from build123d import *

# Parameters (mm, degrees)
SKETCH_2_W                = 72
SKETCH_2_H                = 64
SKETCH_2_R                = 2.25
SKETCH_2_R_2              = 1.75
EXTRUDE_1_DEPTH           = 7
HOLE_WIZARD_1_D           = 4.5
HOLE_WIZARD_1_CBORE_D     = 7.3
HOLE_WIZARD_1_CBORE_DEPTH = 4.2
CUT_EXTRUDE_1_DEPTH       = 2.5


with BuildPart() as part:
    # 草圖2 → 填料-伸長1 (new body)
    with BuildSketch(Plane.XY):
        Rectangle(SKETCH_2_W, SKETCH_2_H)
        with Locations((-18, 18)):
            Circle(SKETCH_2_R, mode=Mode.SUBTRACT)
        with Locations((-31, 26)):
            Circle(SKETCH_2_R_2, mode=Mode.SUBTRACT)
        with Locations((18, 18)):
            Circle(SKETCH_2_R, mode=Mode.SUBTRACT)
        with Locations((18, -18)):
            Circle(SKETCH_2_R, mode=Mode.SUBTRACT)
        with Locations((-18, -18)):
            Circle(SKETCH_2_R, mode=Mode.SUBTRACT)
        with Locations((31, 26)):
            Circle(SKETCH_2_R_2, mode=Mode.SUBTRACT)
        with Locations((31, -26)):
            Circle(SKETCH_2_R_2, mode=Mode.SUBTRACT)
        with Locations((-31, -26)):
            Circle(SKETCH_2_R_2, mode=Mode.SUBTRACT)
    extrude(amount=EXTRUDE_1_DEPTH)

    # 鑽孔1 (through all)
    with Locations(Plane(origin=(-18, 18, 7), x_dir=(1, 0, 0), z_dir=(0, 0, 1))):
        with Locations((0, 0), (36, 0), (36, -36), (0, -36)):
            CounterBoreHole(HOLE_WIZARD_1_D / 2, HOLE_WIZARD_1_CBORE_D / 2, HOLE_WIZARD_1_CBORE_DEPTH)

    # 草圖4 → 除料-伸長1 (cut)
    with BuildSketch(Plane(origin=(0, 0, 0), x_dir=(-1, 0, 0), z_dir=(0, 0, -1))):
        Polygon((-27.709103466, 26), (-29.354551733, 28.85), (-32.645448267, 28.85), (-34.290896534, 26), (-32.645448267, 23.15), (-29.354551733, 23.15), align=None)
        Polygon((29.354551733, 23.15), (27.709103466, 26), (29.354551733, 28.85), (32.645448267, 28.85), (34.290896534, 26), (32.645448267, 23.15), align=None)
        Polygon((27.709103466, -26), (29.354551733, -28.85), (32.645448267, -28.85), (34.290896534, -26), (32.645448267, -23.15), (29.354551733, -23.15), align=None)
        Polygon((-29.354551733, -23.15), (-27.709103466, -26), (-29.354551733, -28.85), (-32.645448267, -28.85), (-34.290896534, -26), (-32.645448267, -23.15), align=None)
    extrude(amount=-CUT_EXTRUDE_1_DEPTH, mode=Mode.SUBTRACT)


solid = part.part
The model under review builds one solid part; all positions refer to its coordinate system, in mm. A direction names the side the tool comes from. Round coordinates to 2 decimals unless told otherwise and drop trailing zeros. Write each loop counter-clockwise with the first axis right and the second up, starting at its lowest first coordinate (ties: lowest second). Pieces come first, ordered by that corner, then holes. Notation, with made-up numbers: (75, -17.5) -> (89, -17.5) arc R15 ccw to (89, -1.5) -> close; hole circle Ø8 at (61.5, 3). An arc over 180 degrees is marked (long way). Answer as a JSON object with one key per item and string values.
1. We need section B-B on x = 31. State the section outline as (y, z) points.
Results found:
{"outline": "(-32, 0) -> (-28.85, 0) -> (-28.85, 2.5) -> (-27.75, 2.5) -> (-27.75, 7) -> (-32, 7) -> close; (-24.25, 2.5) -> (-23.15, 2.5) -> (-23.15, 0) -> (23.15, 0) -> (23.15, 2.5) -> (24.25, 2.5) -> (24.25, 7) -> (-24.25, 7) -> close; (27.75, 2.5) -> (28.85, 2.5) -> (28.85, 0) -> (32, 0) -> (32, 7) -> (27.75, 7) -> close"}
2. The part is to be moulded in two halves that separate along Y. For faces 1 (the face through (-1, 0, 0)), 2 (the face through (29.71, -24.82, 4.72)), say which applies: pulls with the +Y half, pulls with the -Y half, needs draft (parallel to the pull), parting line crosses it, or undercut.
Results found:
{"face 1": "needs draft", "face 2": "undercut"}
3. To check wall thickness, follow line 1 along Y through (x, z) = (18, 5); line 2 along Y through (x, z) = (-31, 5.35); line 3 along X through (y, z) = (-27, 5). State the ranges of each line that lie inside material, in increasing order.
Results found:
{"line 1": "y = -32 to -21.65, -14.35 to 14.35, 21.65 to 32", "line 2": "y = -32 to -27.75, -24.25 to 24.25, 27.75 to 32", "line 3": "x = -36 to -32.44, -29.56 to 29.56, 32.44 to 36"}
4. We need section C-C on z = 1. State how many separate pieces and enclosed holes the cut face has, and give its area (3 significant figures).
Results found:
{"separate pieces": "1", "enclosed holes": "8", "area": "4,430 mm^2"}
5. Clearance check with flat-ended pins moving along their axes: pin 1 (5 mm diameter, centred on x = -18, y = -18, fed in from +Z); pin 2 (2 mm diameter, centred on x = -17.5, y = -18.5, fed in from +Z); pin 3 (4.5 mm diameter, centred on x = -31, y = -26, fed in from -Z). State where each tip first meets the part, or that it passes through.
Results found:
{"pin 1": "stops at z = 2.8", "pin 2": "passes through", "pin 3": "stops at z = 2.5"}
6. We need section A-A on y = -18. State the section outline as (x, z) points, and give its area (3 significant figures).
Results found:
{"outline": "(-36, 0) -> (-20.25, 0) -> (-20.25, 2.8) -> (-21.65, 2.8) -> (-21.65, 7) -> (-36, 7) -> close; (-15.75, 0) -> (15.75, 0) -> (15.75, 2.8) -> (14.35, 2.8) -> (14.35, 7) -> (-14.35, 7) -> (-14.35, 2.8) -> (-15.75, 2.8) -> close; (20.25, 0) -> (36, 0) -> (36, 7) -> (21.65, 7) -> (21.65, 2.8) -> (20.25, 2.8) -> close", "area": "417 mm^2"}
7. Machinability: for faces 3 (the face through (19.038, 16.004, 1.38)), 4 (the face through (16, 16, 2.8)), 5 (the face through (31, 28.85, 1)), which of the approach directions +Z, -Z, +X, -X, +Y, -Y give a long, thin tool a straight path to every point of the face, cutting with its end or side? Answer none if there is none.
Results found:
{"face 3": "+Z, -Z", "face 4": "+Z", "face 5": "-Z"}
